from build123d import *

# Parameters (mm, degrees)
SKETCH1_W           = 25.4
SKETCH1_H           = 57.15
BOSS_EXTRUDE1_DEPTH = 1.5875
SKETCH2_W           = 25.4
SKETCH2_H           = 25.4
BOSS_EXTRUDE2_DEPTH = 1.5875
SKETCH3_R           = 3.302
CUT_EXTRUDE1_DEPTH  = 68.501425911
FILLET1_R           = 6.35


with BuildPart() as part:
    # Sketch1 → Boss-Extrude1 (new body)
    with BuildSketch(Plane(origin=(0, 0, 0), x_dir=(1, 0, 0), z_dir=(0, 1, 0))):
        with Locations((12.7, 28.575)):
            Rectangle(SKETCH1_W, SKETCH1_H)
    extrude(amount=BOSS_EXTRUDE1_DEPTH)

    # Sketch2 → Boss-Extrude2 (add)
    with BuildSketch(Plane(origin=(0, 0, -57.15), x_dir=(-1, 0, 0), z_dir=(0, 0, -1))):
        with Locations((-12.7, 12.7)):
            Rectangle(SKETCH2_W, SKETCH2_H)
    extrude(amount=BOSS_EXTRUDE2_DEPTH)

    # Sketch3 → Cut-Extrude1 (cut, through all)
    with BuildSketch(Plane.XY.offset(-57.15)):
        with Locations((12.7, 14.2875)):
            Circle(SKETCH3_R)
    extrude(amount=-CUT_EXTRUDE1_DEPTH, mode=Mode.SUBTRACT)

    # Fillet1
    fillet1_edges = [part.edges().sort_by_distance(p)[0] for p in [
        (25.4, 25.4, -57.94375),
        (0, 25.4, -57.94375),
    ]]
    fillet(fillet1_edges, radius=FILLET1_R)


solid = part.part
Verification items for the finished model (mm, model axes). A direction names the side the tool comes from. Coordinates: 2 decimals unless noted, no trailing zeros. Order: outer loops, then holes, each group sorted by start corner. A loop starts at its lowest first (then second) coordinate and runs counter-clockwise, first axis right, second up. Notation, with made-up numbers: M 83.25,-4 L 121.25,-4 A21 ccw 121.25,2 Z; hole C 87.5,29.5 d9. An arc over 180 degrees is marked long. One line per item, written item: value. Start each with the question number.
Item 1: Sectioned sample at B-B on y = 12. Record the cut outline in (x, z).
Item 2: Thickness scan on probe 1 along Y at (x, z) = (12.7, -57.75); probe 2 along Y at (x, z) = (16.25, -11.5); probe 3 along Z at (x, y) = (21, 17.5). Record the ranges inside material, lowest first.
Item 3: Mould release check, pull along X, two halves, no side actions. Record for faces 3 (the cylindrical face through (11.984, 11.064, -57.933)), 4 (the flat face through (13, 1.588, -29)), 5 (the flat face through (0, 1, -38)): pulls with the +X half, pulls with the -X half, needs draft (parallel to the pull), parting line crosses it, or undercut.
Item 4: Depth check by flat-ended pin: P1, Ø5, axis at x = 8, z = -52.5, coming from the +Y side; P2, Ø3, axis at x = 6, y = 11.5, coming from the +Z side. Enter the tip coordinate at first touch or a pass-through.
Item 5: Sectioned sample at C-C on x = 22. Record the cut outline in (y, z), then the cut area to 3 significant figures.
Item 6: Sectioned sample at D-D on z = -32.5. Record the cut outline in (x, y), then the cut area to 3 significant figures.
Item 7: Access from +Z, -Z, +X, -X, +Y, -Y to the whole of each face (thin tool, end or side, straight path). Record for faces 1 (the flat face through (13, 0, -29)), 2 (the flat face through (10, 11, -57.15)).
Item 8: Sectioned sample at A-A on x = 12.7. Record the cut outline in (y, z).
Calculated:
1. outline: M 0,-58.74 L 10.32,-58.74 L 10.32,-57.15 L 0,-57.15 Z; M 15.08,-58.74 L 25.4,-58.74 L 25.4,-57.15 L 15.08,-57.15 Z
2. probe 1: 0 to 10.99, 17.59 to 25.4
2. probe 2: 0 to 1.59
2. probe 3: -58.74 to -57.15
3. face 3: undercut
3. face 4: needs draft
3. face 5: pulls with the -X half
4. P1: y = 1.59
4. P2: z = -57.15
5. outline: M 0,-58.74 L 24.67,-58.74 L 24.67,-57.15 L 1.59,-57.15 L 1.59,0 L 0,0 Z
5. area: 130 mm^2
6. outline: M 0,0 L 25.4,0 L 25.4,1.59 L 0,1.59 Z
6. area: 40.3 mm^2
7. face 1: +Z, -Z, +X, -X, -Y
7. face 2: +Z, +X, -X, +Y
8. outline: M 0,-58.74 L 10.99,-58.74 L 10.99,-57.15 L 1.59,-57.15 L 1.59,0 L 0,0 Z; M 17.59,-58.74 L 25.4,-58.74 L 25.4,-57.15 L 17.59,-57.15 Z
